Autodesk Inventor part; units mm, degrees
ref_plane "YZ Plane" through (0, 0, 0) normal (1, 0, 0) x (0, 1, 0)
ref_plane "XZ Plane" through (0, 0, 0) normal (0, 1, 0) x (-1, 0, 0)
ref_plane "XY Plane" through (0, 0, 0) normal (0, 0, 1) x (1, 0, 0)
ref_plane "Arbeitsebene1" through (-858.9244, 0, 0) normal (0, 0, 1) x (1, 0, 0)
sketch "Skizze2" plane through (-858.9244, 0, 0) normal (0, 0, 1) x (1, 0, 0)
  line L0 (-100.0619, 347.3197) -> (439.9381, 347.3197)
  line L1 (439.9381, 347.3197) -> (439.9381, -192.6803)
  line L2 (439.9381, -192.6803) -> (-100.0619, -192.6803)
  line L3 (-100.0619, -192.6803) -> (-100.0619, 347.3197)
  point P0 (858.9244, 0)
  dimension "d5" = 540
  dimension "d6" = 540
extrude "Extrusion2" add sketch "Skizze2" along normal blind 18
chamfer "Fase2" distance 18 angle 45 4 edges at (-688.9863, -192.6803, 0) (-418.9863, 77.3197, 0) (-958.9863, 77.3197, 0) (-688.9863, 347.3197, 0)
sketch "Skizze3" plane through (-858.9244, 0, 0) normal (0, 0, -1) x (-1, 0, 0)
  line L0 (58.0619, -154.6803) -> (11.0619, -154.6803)
  line L1 (7.0619, -150.6803) -> (7.0619, -48.6803)
  line L2 (11.0619, -44.6803) -> (58.0619, -44.6803)
  line L3 (62.0619, -48.6803) -> (62.0619, -150.6803)
  line L4 (82.0619, -174.6803) -> (-421.9381, -174.6803)
  line L5 (82.0619, 329.3197) -> (82.0619, -174.6803)
  arc A0 (58.0619, -154.6803) -> (62.0619, -150.6803) centre (58.0619, -150.6803) ccw
  arc A1 (7.0619, -150.6803) -> (11.0619, -154.6803) centre (11.0619, -150.6803) ccw
  arc A2 (11.0619, -44.6803) -> (7.0619, -48.6803) centre (11.0619, -48.6803) ccw
  arc A3 (62.0619, -48.6803) -> (58.0619, -44.6803) centre (58.0619, -48.6803) ccw
  point P0 (-858.9244, 0)
  point P1 (7.0619, -44.6803)
  point P2 (7.0619, -154.6803)
  point P3 (62.0619, -44.6803)
  dimension "d12" = 55
  dimension "d13" = 110
  dimension "d14" = 20
  dimension "d15" = 20
  dimension "d16" = 4
extrude "Extrusion3" cut sketch "Skizze3" against normal blind 15
properties part number "Sitzfläche"
For this review, take the finished solid that the model builds, in its own axes (mm). A direction names the side the tool comes from. Round coordinates to 2 decimals unless told otherwise and drop trailing zeros. Loops run counter-clockwise (first coordinate to the right, second up) from the corner with the lowest first, then second, coordinate; pieces in that order, holes last. Notation, with made-up numbers: (9, 27.25) - (52, 27.25) arc R7 cw to (52, 36.25) - close; hole circle Ø4 at (39, 11.25). An arc over 180 degrees is marked (long way). Use one line per item in the form item = value.
Item 1: Consider section B-B on z = 6. Write out the cut boundary in (x, y), then the cut area to 3 significant figures.
Answers:
outline = (-946.99, -180.68) - (-430.99, -180.68) - (-430.99, 335.32) - (-946.99, 335.32) - close; hole (-920.99, -150.68) arc R4 ccw to (-916.99, -154.68) - (-869.99, -154.68) arc R4 ccw to (-865.99, -150.68) - (-865.99, -48.68) arc R4 ccw to (-869.99, -44.68) - (-916.99, -44.68) arc R4 ccw to (-920.99, -48.68) - close
area = 260,000 mm^2
Item 2: Mouldability with a two-part tool opening along X and no side actions: class faces 1 (the flat face through (-865.986, -100, 7)), 2 (the flat face through (-894, -154.68, 7)), 3 (the flat face through (-428.112, 73.54, 8.874)), 4 (the flat face through (-692.77, -183.55, 8.87)) as +X half, -X half, draft (parallel to the pull), parting line (faces both ways), or undercut.
Answers:
face_1 = undercut
face_2 = undercut
face_3 = +X half
face_4 = draft
Item 3: Tool access review of faces 5 (the flat face through (-893, -99, 15)), 6 (the flat face through (-949.861, 81.1, 8.874)): name each direction out of +Z, -Z, +X, -X, +Y, -Y from which nothing blocks a thin tool from reaching the whole face with its end or side.
Answers:
face_5 = -Z
face_6 = -Z, -X, +Y, -Y
Item 4: For line 1 (X direction, y = -84, z = 13); line 2 (X direction, y = -128, z = 6.5); line 3 (Y direction, x = -565.5, z = 13.5), list the stretches that pass through material, from the lowest coordinate up.
Answers:
line_1 = -953.99 to -920.99, -865.99 to -423.99
line_2 = -947.49 to -920.99, -865.99 to -430.49
line_3 = -188.18 to 342.82
Item 5: Clearance check with flat-ended pins moving along their axes: P1, Ø4, axis at x = -858, z = 5, coming from the +Y side; P2, Ø1.5, axis at x = -547.5, z = 2.5, coming from the -Y side; P3, Ø5, axis at x = -577, z = 5.5, coming from the -Y side; P4, Ø4, axis at x = -655.5, y = 289.5, coming from the -Z side. State where each tip first meets the part, or that it passes through.
Answers:
P1 = 336.32
P2 = -177.93
P3 = -182.68
P4 = 0
